Autodesk Inventor part; units mm, degrees
ref_plane "YZ Plane" through (0, 0, 0) normal (1, 0, 0) x (0, 1, 0)
ref_plane "XZ Plane" through (0, 0, 0) normal (0, 1, 0) x (-1, 0, 0)
ref_plane "XY Plane" through (0, 0, 0) normal (0, 0, 1) x (1, 0, 0)
sketch "Skizze1" plane through (0, 0, 0) normal (0, 0, 1) x (1, 0, 0)
  line L0 (-245, 0) -> (245, 0)
  line L1 (0, -245) -> (0, 245)
  line L2 (175, 7.5) -> (175, -7.5)
  line L3 (-175, -7.5) -> (-175, 7.5)
  line L4 (-7.5, 175) -> (7.5, 175)
  line L5 (7.5, -175) -> (-7.5, -175)
  circle A0 centre (0, 170) radius 2.5
  circle A1 centre (0, -170) radius 2.5
  circle A2 centre (-170, 0) radius 2.5
  circle A3 centre (170, 0) radius 2.5
  circle A4 centre (0, 0) radius 165
  line L6 (7.5, 175) -> (7.5, 164.8295)
  line L7 (-7.5, 164.8295) -> (-7.5, 175)
  line L8 (-175, 7.5) -> (-164.8295, 7.5)
  line L9 (-164.8295, -7.5) -> (-175, -7.5)
  line L10 (175, -7.5) -> (164.8295, -7.5)
  line L11 (164.8295, 7.5) -> (175, 7.5)
  line L12 (7.5, -164.8295) -> (7.5, -175)
  line L13 (-7.5, -175) -> (-7.5, -164.8295)
  circle A5 centre (0, 0) radius 162.5
  dimension "d12" = 330
  dimension "d2" = 350
  dimension "d3" = 350
  dimension "d4" = 5
  dimension "d5" = 5
  dimension "d6" = 5
  dimension "d7" = 5
  dimension "d8" = 5
  dimension "d9" = 5
  dimension "d10" = 5
  dimension "d11" = 5
  dimension "d13" = 325
extrude "Extrusion1" add sketch "Skizze1" along normal blind 3 contours A4 L11 L2 L0 A3 | L0 A3 L2 L10 A4 | A4 L7 L4 L1 A0 | L1 A0 L4 L6 A4 | A4 L12 L5 L1 A1 | L1 A1 L5 L13 A4 | A4 L9 L3 L0 A2 | L0 A2 L3 L8 A4
sketch "Skizze2" plane through (0, 0, 0) normal (0, 0, 1) x (1, 0, 0)
  line L0 (-231, 0) -> (231, 0)
  line L1 (0, -231) -> (0, 231)
  circle A0 centre (0, 0) radius 165
  circle A1 centre (0, 0) radius 162.5
  dimension "d16" = 330
  dimension "d17" = 325
extrude "Extrusion2" add sketch "Skizze2" along normal blind 50
sketch "Skizze3" plane through (0, 0, 50) normal (0, 0, 1) x (1, 0, 0)
  circle A0 centre (0, 0) radius 162.5
  dimension "d20" = 325
extrude "Extrusion3" cut sketch "Skizze3" against normal blind 50
sketch "Skizze5" plane through (0, 0, 50) normal (0, 0, 1) x (1, 0, 0)
  line L0 (-249.0675, 0) -> (269.4048, 0)
  line L1 (0, -269.4048) -> (0, 249.0675)
  line L2 (-2.5, 165) -> (2.5, 165)
  line L3 (2.5, 165) -> (2.5, -165)
  line L4 (2.5, -165) -> (-2.5, -165)
  line L5 (-2.5, -165) -> (-2.5, 165)
  line L6 (-165, 2.5) -> (165, 2.5)
  line L7 (165, 2.5) -> (165, -2.5)
  line L8 (165, -2.5) -> (-165, -2.5)
  line L9 (-165, -2.5) -> (-165, 2.5)
  circle A0 centre (0, 0) radius 165
  circle A1 centre (0, 0) radius 162.5
  line L10 (-80.3255, 144.1278) -> (0, 5)
  line L11 (-84.6556, 141.6278) -> (-6.8301, 6.8301)
  line L12 (-6.8301, 6.8301) -> (-141.6278, 84.6556)
  line L13 (-9.3301, 2.5) -> (-144.1278, 80.3255)
  line L14 (0, 5) -> (80.3255, 144.1278)
  line L15 (6.8301, 6.8301) -> (84.6556, 141.6278)
  line L16 (9.3301, 2.5) -> (144.1278, 80.3255)
  line L17 (6.8301, 6.8301) -> (141.6278, 84.6556)
  line L18 (-144.1278, -80.3255) -> (-9.3301, -2.5)
  line L19 (-141.6278, -84.6556) -> (-6.8301, -6.8301)
  line L20 (-80.3255, -144.1278) -> (-2.5, -9.3301)
  line L21 (-84.6556, -141.6278) -> (-6.8301, -6.8301)
  arc A2 (7.5, -164.8295) -> (164.8295, -7.5) centre (0, 0) ccw
  line L22 (2.5, -9.3301) -> (80.3255, -144.1278)
  line L23 (6.8301, -6.8301) -> (141.6278, -84.6556)
  line L24 (144.1278, -80.3255) -> (9.3301, -2.5)
  line L25 (84.6556, -141.6278) -> (6.8301, -6.8301)
  line L26 (141.6278, -84.6556) -> (144.1278, -80.3255)
  line L27 (141.6278, 84.6556) -> (144.1278, 80.3255)
  line L28 (80.3255, 144.1278) -> (84.6556, 141.6278)
  line L29 (-84.6556, 141.6278) -> (-80.3255, 144.1278)
  line L30 (-144.1278, 80.3255) -> (-141.6278, 84.6556)
  line L31 (-141.6278, -84.6556) -> (-144.1278, -80.3255)
  line L32 (-80.3255, -144.1278) -> (-84.6556, -141.6278)
  point P0 (-142.8942, 82.5)
  point P1 (79.0753, -141.9625)
  point P2 (83.4054, -139.4625)
  point P3 (139.4625, -83.4054)
  point P4 (141.9625, -79.0753)
  point P5 (141.9625, 79.0753)
  point P6 (139.4625, 83.4054)
  point P7 (83.4054, 139.4625)
  point P8 (79.0753, 141.9625)
  point P9 (2.5, 9.3301)
  point P10 (-2.5, 9.3301)
  point P11 (-79.0753, 141.9625)
  point P12 (-83.4054, 139.4625)
  point P13 (-139.4625, 83.4054)
  point P14 (-141.9625, 79.0753)
  point P15 (-141.9625, -79.0753)
  point P16 (-139.4625, -83.4054)
  point P17 (-83.4054, -139.4625)
  point P18 (-79.0753, -141.9625)
  dimension "d23" = 5
  dimension "d24" = 5
  dimension "d25" = 330
  dimension "d26" = 330
  dimension "d30" = 5
  dimension "d34" = 5
  dimension "d37" = 5
  dimension "d38" = 5
  dimension "d43" = 5
  dimension "d44" = 5
  dimension "d46" = 5
extrude "Extrusion4" add sketch "Skizze5" along normal blind 3 contours A1 L6 A0 L0 | A1 L8 L3 L0 | L0 L3 L6 A1 | L0 A0 L8 A1 | A0 L6 L7 | L7 L8 A0 | L3 L8 L1 L0 | L0 L1 L6 L3 | L1 L8 L5 L0 | L0 L5 L6 L1 | L6 L1 L14 L3 | L3 L14 A1 L15 L17 L16 L6 | L8 L24 A1 L23 L25 L22 L3 | L3 A1 L1 L8 | L5 L8 A1 L0 | L0 A1 L6 L5 | L1 A1 L5 L8 | L6 L5 L10 L1 | L14 L1 A1 L3 | A1 L8 A0 L0 | L0 A0 L6 A1 | L5 L20 A1 L21 L19 L18 L8 | L6 L13 A1 L12 L11 L10 L5 | A1 L3 A0 L1 | L1 A0 L5 A1 | L10 L5 A1 L1 | A1 L1 A0 L3 | A0 L8 L9 | L9 L6 A0 | A0 L3 L4 | L4 L5 A0 | A1 L5 A0 L1 | A0 L2 L3 | A0 L5 L2
sketch "Skizze6" plane through (0, 0, 53) normal (0, 0, 1) x (1, 0, 0)
  circle A0 centre (0, 0) radius 50
  dimension "d49" = 100
extrude "Extrusion5" add sketch "Skizze6" along normal blind 15 draft -45 and the other way blind 3
sketch "Skizze7" plane through (0, 0, 50) normal (0, 0, -1) x (-1, 0, 0)
  circle A0 centre (0, 0) radius 5
  dimension "d54" = 10
extrude "Extrusion6" cut sketch "Skizze7" against normal blind 10
properties part number "Ventilator"
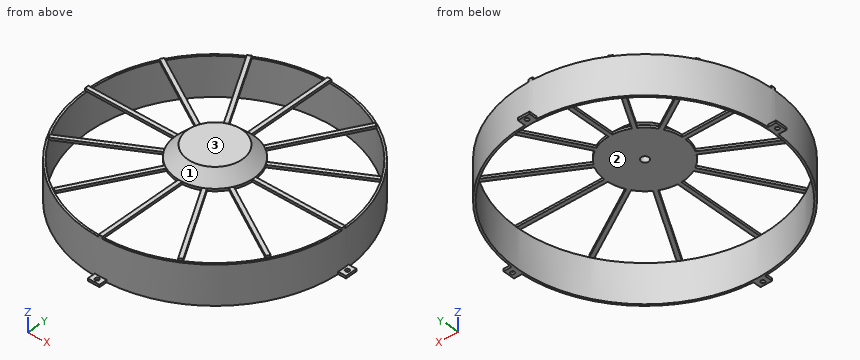
For this review, take the finished solid that the model builds, in its own axes (mm). Face numbers are marked on the shaded views. Round coordinates to 2 decimals unless told otherwise and drop trailing zeros. Write each loop counter-clockwise with the first axis right and the second up, starting at its lowest first coordinate (ties: lowest second). Pieces come first, ordered by that corner, then holes.
1) Insertion check: pin 1 Ø18 at (x, y) = (-87, 39) entering from +Z; pin 2 Ø3.5 at (x, z) = (102, 51) entering from -Y; pin 3 Ø0.9 at (y, z) = (118, 51.5) entering from +X. Each pin has a flat end and moves straight along its axis. Give the tip position at first contact, or say it passes through.
Answer below:
pin 1: stops at z = 53
pin 2: stops at y = -130.81
pin 3: stops at x = 71.27
2) Take a section at C-C on y = -119. Give the boundary of the cut face in (x, z).
Answer below:
outline: (-114.3, 0) - (-110.66, 0) - (-110.66, 50) - (-114.3, 50) - close; (-71.59, 50) - (-65.82, 50) - (-65.82, 53) - (-71.59, 53) - close; (-2.5, 50) - (2.5, 50) - (2.5, 53) - (-2.5, 53) - close; (65.82, 50) - (71.59, 50) - (71.59, 53) - (65.82, 53) - close; (110.66, 0) - (114.3, 0) - (114.3, 50) - (110.66, 50) - close
3) For line 1 along X through (y, z) = (0, 2.15); line 2 along Y through (x, z) = (0, 21.5), list the stretches that pass through material, from the lowest coordinate up.
Answer below:
line 1: x = -175 to -172.5, -167.5 to -162.5, 162.5 to 167.5, 172.5 to 175
line 2: y = -165 to -162.5, 162.5 to 165
4) Take a section at D-D on y = 57. Give the boundary of the cut face in (x, z).
Answer below:
outline: (-154.84, 0) - (-152.18, 0) - (-152.18, 50) - (-154.84, 50) - close; (-103.73, 50) - (-93.73, 50) - (-93.73, 53) - (-103.73, 53) - close; (-35.8, 50) - (-30.02, 50) - (-30.02, 53) - (-35.8, 53) - close; (-2.5, 50) - (2.5, 50) - (2.5, 53) - (-2.5, 53) - close; (30.02, 50) - (35.8, 50) - (35.8, 53) - (30.02, 53) - close; (93.73, 50) - (103.73, 50) - (103.73, 53) - (93.73, 53) - close; (152.18, 0) - (154.84, 0) - (154.84, 50) - (152.18, 50) - close
5) Mouldability with a two-part tool opening along Y and no side actions: class the marked faces 1, 2 and 3 as +Y half, -Y half, draft (parallel to the pull), parting line (faces both ways), or undercut.
Answer below:
face 1: parting line
face 2: undercut
face 3: draft
6) Take a section at A-A on y = -63. Give the boundary of the cut face in (x, z), then the cut area to 3 significant figures.
Answer below:
outline: (-152.5, 0) - (-149.79, 0) - (-149.79, 50) - (-152.5, 50) - close; (-114.12, 50) - (-104.12, 50) - (-104.12, 53) - (-114.12, 53) - close; (-39.26, 50) - (-33.49, 50) - (-33.49, 53) - (-39.26, 53) - close; (-2.5, 50) - (2.5, 50) - (2.5, 53) - (-2.5, 53) - close; (33.49, 50) - (39.26, 50) - (39.26, 53) - (33.49, 53) - close; (104.12, 50) - (114.12, 50) - (114.12, 53) - (104.12, 53) - close; (149.79, 0) - (152.5, 0) - (152.5, 50) - (149.79, 50) - close
area: 380 mm2
7) Take a section at B-B on z = 21.5. Give the boundary of the cut face in (x, y).
Answer below:
outline: circle Ø330 at (0, 0); hole circle Ø325 at (0, 0)
